```python
from build123d import *

# Parameters (mm, degrees)
SKETCH1_W                = 37
SKETCH1_H                = 22.4
BOSS_EXTRUDE1_DEPTH      = 18.6
BOSS_EXTRUDE2_DEPTH      = 30
BOSS_EXTRUDE3_DEPTH      = 8.7
BOSS_EXTRUDE3_DEPTH_BACK = 27.3
SKETCH3_R                = 2.5
SKETCH4_R                = 1.5
CUT_EXTRUDE1_DEPTH       = 18.6
FILLET2_R                = 2.5


with BuildPart() as part:
    # Sketch1 → Boss-Extrude1 (new body)
    with BuildSketch(Plane.XY):
        with Locations((18.5, 11.2)):
            Rectangle(SKETCH1_W, SKETCH1_H)
    extrude(amount=BOSS_EXTRUDE1_DEPTH)

    # Sketch2 → Boss-Extrude2 (add)
    with BuildSketch(Plane.ZY):
        with BuildLine():
            Line((0, 17.440993511), (0, 4.959006489))
            ThreePointArc((0, 4.959006489), (9.3, 0), (18.6, 4.959006489))
            Line((18.6, 4.959006489), (18.6, 17.440993511))
            ThreePointArc((18.6, 17.440993511), (9.3, 22.4), (0, 17.440993511))
        make_face()
    extrude(amount=BOSS_EXTRUDE2_DEPTH)

    # Sketch3 → Boss-Extrude3 (add, two sides: drawn at the far end of the back side and taken through both)
    with BuildSketch(Plane.XY.offset(18.6).offset(-BOSS_EXTRUDE3_DEPTH_BACK)):
        with Locations((25.5, 11.2)):
            Circle(SKETCH3_R)
    extrude(amount=BOSS_EXTRUDE3_DEPTH + BOSS_EXTRUDE3_DEPTH_BACK)

    # Sketch4 → Cut-Extrude1 (cut)
    with BuildSketch(Plane.XY.offset(18.6)):
        with Locations((5.65, 20)):
            Circle(SKETCH4_R)
        with Locations((5.65, 2.4)):
            Circle(SKETCH4_R)
    extrude(amount=-CUT_EXTRUDE1_DEPTH, mode=Mode.SUBTRACT)

    # Fillet2
    fillet2_edges = [part.edges().sort_by_distance(p)[0] for p in [
        (37, 22.4, 9.3),
        (37, 0, 9.3),
    ]]
    fillet(fillet2_edges, radius=FILLET2_R)


solid = part.part
```
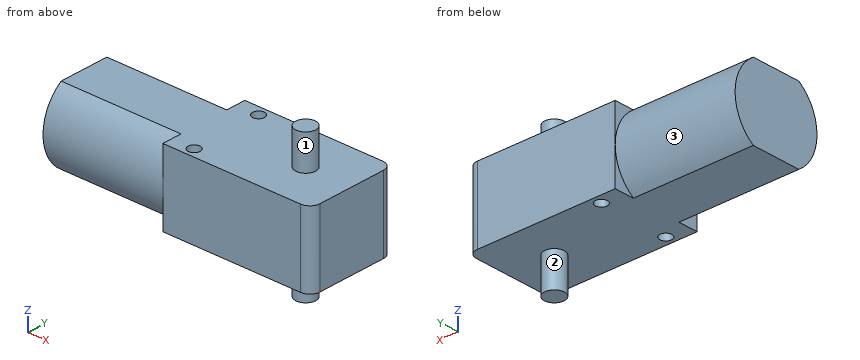
Model file for the job. Use its own axes, mm. Face numbers are marked on the shaded views. A direction names the side the tool comes from. Coordinates: 2 decimals unless noted, no trailing zeros. Loops run counter-clockwise (first coordinate to the right, second up) from the corner with the lowest first, then second, coordinate; pieces in that order, holes last. Notation, with made-up numbers: (-33, 61) -> (9, 61) arc R11 cw to (9, 66) -> close; hole circle Ø10 at (-10.75, 23). An arc over 180 degrees is marked (long way). Answer as a JSON object with one key per item and string values.
Q1. Cut at D-D (z = 11.5). List the corners of the cut face in (x, y), and give its area (3 significant figures).
Report:
{"outline": "(-30, 0.22) -> (0, 0.22) -> (0, 0) -> (34.5, 0) arc R2.5 ccw to (37, 2.5) -> (37, 19.9) arc R2.5 ccw to (34.5, 22.4) -> (0, 22.4) -> (0, 22.18) -> (-30, 22.18) -> close; hole circle Ø3 at (5.65, 2.4); hole circle Ø3 at (5.65, 20)", "area": "1,470 mm2"}
Q2. Cut at B-B (y = 11.2). List the corners of the cut face in (x, z).
Report:
{"outline": "(-30, 0) -> (23, 0) -> (23, -8.7) -> (28, -8.7) -> (28, 0) -> (37, 0) -> (37, 18.6) -> (28, 18.6) -> (28, 27.3) -> (23, 27.3) -> (23, 18.6) -> (-30, 18.6) -> close"}
Q3. Flat gauge pins, fed straight in: P1, Ø5, axis at x = 5.65, y = 2.4, coming from the -Z side; P2, Ø10, axis at x = -17.5, z = 0, coming from the +Y side; P3, Ø6.5, axis at x = 2, y = 17, coming from the +Z side. Where does each tip first touch, or does it go through?
Report:
{"P1": "stops at z = 0", "P2": "stops at y = 21.54", "P3": "stops at z = 18.6"}
Q4. Cut at C-C (x = 24). List the corners of the cut face in (y, z), and give its area (3 significant figures).
Report:
{"outline": "(0, 0) -> (9.2, 0) -> (9.2, -8.7) -> (13.2, -8.7) -> (13.2, 0) -> (22.4, 0) -> (22.4, 18.6) -> (13.2, 18.6) -> (13.2, 27.3) -> (9.2, 27.3) -> (9.2, 18.6) -> (0, 18.6) -> close", "area": "486 mm2"}
Q5. Probe probe 1 along Y at (x, z) = (5.65, 11.5); probe 2 along Z at (x, y) = (17, 7); probe 3 along X at (y, z) = (19.5, 5). List the from-to ranges inside material, lowest first.
Report:
{"probe 1": "y = 0 to 0.9, 3.9 to 18.5, 21.5 to 22.4", "probe 2": "z = 0 to 18.6", "probe 3": "x = -30 to 4.24, 7.06 to 37"}
Q6. 3-axis set-ups, long thin cutter, end or side, ignore diameter. For the marked faces 1, 2 and 3: which of +Z, -Z, +X, -X, +Y, -Y reach the whole face in a straight line?
Report:
{"face 1": "+Z", "face 2": "-Z", "face 3": "-X, +Y"}
Q7. Cut at A-A (x = 5.65). List the corners of the cut face in (y, z), and give its area (3 significant figures).
Report:
{"outline": "(0, 0) -> (0.9, 0) -> (0.9, 18.6) -> (0, 18.6) -> close; (3.9, 0) -> (18.5, 0) -> (18.5, 18.6) -> (3.9, 18.6) -> close; (21.5, 0) -> (22.4, 0) -> (22.4, 18.6) -> (21.5, 18.6) -> close", "area": "305 mm2"}
